Check sheet for the drawn part. Datum: minimum x, y, z corner. Units: mm. A direction names the side the tool comes from. Coordinates: 2 decimals unless noted, no trailing zeros. Order: outer loops, then holes, each group sorted by start corner. A loop starts at its lowest first (then second) coordinate and runs counter-clockwise, first axis right, second up.
Q1. Set-up check for the marked faces 1 and 2: record each of +Z, -Z, +X, -X, +Y, -Y from which the full face is reachable in a straight line by a thin tool's end or side.
Q2. Thickness scan on line 1 (X direction, y = 410.5, z = 51); line 2 (Y direction, x = 25.5, z = 15.5); line 3 (Y direction, x = 34.5, z = 8). Record the ranges inside material, lowest first.
Q3. Cross-section at A-A, the plane z = 17. Record the boundary of the cut face in (x, y) (1 decimal).
Q4. Draft check along Y on the marked faces 3, 4 and 5. Enter one of: pulls with the +Y half, pulls with the -Y half, needs draft (parallel to the pull), parting line crosses it, or undercut.
Q5. Cross-section at B-B, the plane y = 41. Record the boundary of the cut face in (x, z).
Q6. Cross-section at C-C, the plane z = 53.5. Record the boundary of the cut face in (x, y) (1 decimal), and give its area (3 significant figures).
Q7. Depth check by flat-ended pin: P1, Ø3, axis at x = 12, z = 49.5, coming from the +Y side (1 decimal); P2, Ø8, axis at x = 26, z = 30.5, coming from the +Y side. Enter the tip coordinate at first touch or a pass-through.
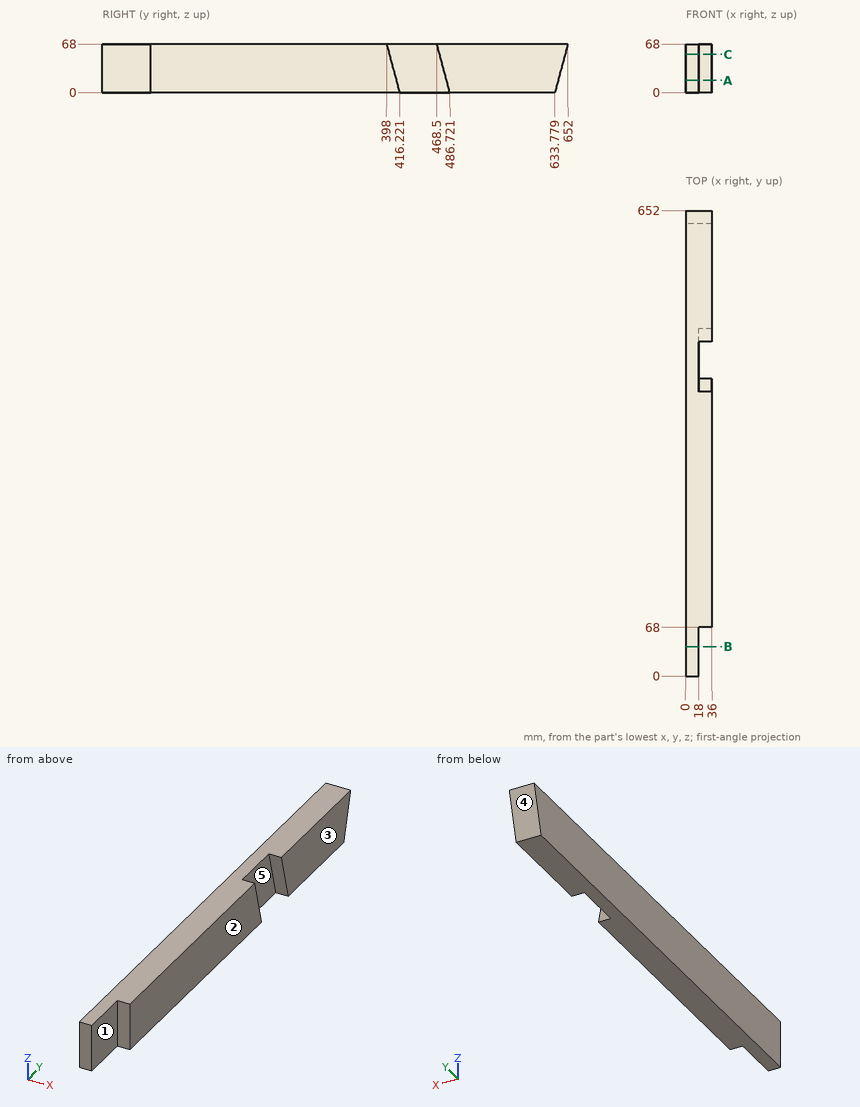
Check values:
1. face 1: +Z, -Z, +X, -Y
1. face 2: +Z, -Z, +X, +Y, -Y
2. line 1: x = 0 to 18
2. line 2: y = 68 to 412.07, 482.57 to 637.93
2. line 3: y = 68 to 414.08, 484.58 to 635.92
3. outline: (0, 0) - (18, 0) - (18, 68) - (36, 68) - (36, 411.7) - (18, 411.7) - (18, 482.2) - (36, 482.2) - (36, 638.3) - (0, 638.3) - close
4. face 3: needs draft
4. face 4: pulls with the +Y half
4. face 5: undercut
5. outline: (0, 0) - (18, 0) - (18, 68) - (0, 68) - close
6. outline: (0, 0) - (18, 0) - (18, 68) - (36, 68) - (36, 401.9) - (18, 401.9) - (18, 472.4) - (36, 472.4) - (36, 648.1) - (0, 648.1) - close
6. area: 20,800 mm2
7. P1: stops at y = 647.4
7. P2: stops at y = 643.02
